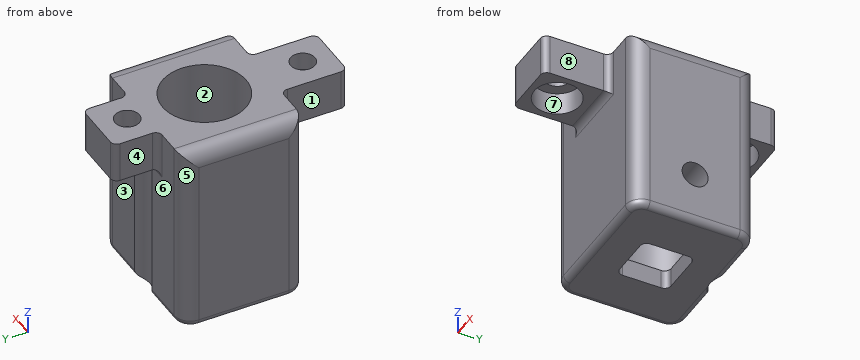
```python
from build123d import *

# Parameters (mm, degrees)
SKETCH1_W                                      = 23
SKETCH1_H                                      = 19
SKETCH1_W_2                                    = 8
SKETCH1_H_2                                    = 8
TOP_DEPTH                                      = 3
SKETCH1_4_W                                    = 23
SKETCH1_4_H                                    = 19
SKETCH1_4_R                                    = 6.5
BODY_DEPTH                                     = 29.83
TABS_START                                     = 23.48
SKETCH1_6_W                                    = 9
SKETCH1_6_H                                    = 7
SKETCH1_6_H_2                                  = 10.3075
TABS_DEPTH                                     = 6.35
F_36_0_1065_DIA_SET_SCREW_D                    = 4.0386
F_36_0_1065_DIA_SET_SCREW_DEPTH                = 4.826
F_36_0_1065_DIA_SET_SCREW_TIP                  = 1.213317848
CBORE_FOR_6_SOCKET_HEAD_CAP_SCREW1_D           = 3.7973
CBORE_FOR_6_SOCKET_HEAD_CAP_SCREW1_CBORE_D     = 7.14502
CBORE_FOR_6_SOCKET_HEAD_CAP_SCREW1_CBORE_DEPTH = 26.9851886
FILLET4_R                                      = 2.5
FILLET5_R                                      = 1


with BuildPart() as part:
    # Sketch1 → Top (new body)
    with BuildSketch(Plane.XY):
        Rectangle(SKETCH1_W, SKETCH1_H)
        Rectangle(SKETCH1_W_2, SKETCH1_H_2, mode=Mode.SUBTRACT)
    extrude(amount=TOP_DEPTH)

    # Sketch1<4> → Body (add)
    with BuildSketch(Plane.XY):
        Rectangle(SKETCH1_4_W, SKETCH1_4_H)
        Circle(SKETCH1_4_R, mode=Mode.SUBTRACT)
    extrude(amount=BODY_DEPTH)

    # Sketch1<6> → Tabs (add)
    with BuildSketch(Plane.XY.offset(TABS_START)):
        with Locations((0, 13)):
            Rectangle(SKETCH1_6_W, SKETCH1_6_H)
        with Locations((0, -14.65375)):
            Rectangle(SKETCH1_6_W, SKETCH1_6_H_2)
    extrude(amount=TABS_DEPTH)

    # #36 (0.1065) Dia. Set Screw
    with Locations(Plane(origin=(11.5, 0, 0), x_dir=(0, 0, -1), z_dir=(1, 0, 0))):
        with Locations((-8, 0)):
            Hole(F_36_0_1065_DIA_SET_SCREW_D / 2, depth=F_36_0_1065_DIA_SET_SCREW_DEPTH)
            with Locations((0, 0, -(F_36_0_1065_DIA_SET_SCREW_DEPTH + F_36_0_1065_DIA_SET_SCREW_TIP / 2))):  # 118° drill point
                Cone(0, F_36_0_1065_DIA_SET_SCREW_D / 2, F_36_0_1065_DIA_SET_SCREW_TIP, mode=Mode.SUBTRACT)

    # CBORE for #6 Socket Head Cap Screw1 (through all)
    with Locations(Plane(origin=(0, 12, 0), x_dir=(-1, 0, 0), z_dir=(0, 0, -1))):
        with Locations((0, 0), (0, -27.3035)):
            CounterBoreHole(CBORE_FOR_6_SOCKET_HEAD_CAP_SCREW1_D / 2, CBORE_FOR_6_SOCKET_HEAD_CAP_SCREW1_CBORE_D / 2, CBORE_FOR_6_SOCKET_HEAD_CAP_SCREW1_CBORE_DEPTH)

    # Fillet4
    fillet4_edges = [part.edges().sort_by_distance(p)[0] for p in [
        (-11.5, 9.5, 14.915),
        (-11.5, -9.5, 14.915),
        (11.5, -9.5, 14.915),
        (11.5, 9.5, 14.915),
        (-11.5, 0, 29.83),
        (11.5, 0, 29.83),
    ]]
    fillet(fillet4_edges, radius=FILLET4_R)

    # Fillet5
    fillet5_edges = [part.edges().sort_by_distance(p)[0] for p in [
        (-11.5, 0, 0),
        (11.5, 0, 0),
        (0, -9.5, 0),
        (-5.776012118, 9.5, 0),
        (10.767766953, 8.767766953, 0),
        (10.767766953, -8.767766953, 0),
        (-10.767766953, -8.767766953, 0),
        (-10.767766953, 8.767766953, 0),
        (-4, 4, 1.5),
        (-4, -4, 1.5),
        (4, -4, 1.5),
        (4, 4, 1.5),
        (-4.5, 16.5, 26.655),
        (-3.526012118, 9.5, 23.48),
        (-4.5, 9.5, 26.655),
        (4.5, 9.5, 26.655),
        (4.5, 16.5, 26.655),
        (4.5, -9.5, 26.655),
        (-4.5, -9.5, 26.655),
        (-4.5, -19.8075, 26.655),
        (4.5, -19.8075, 26.655),
        (0, -9.5, 23.48),
        (5.776012118, 9.5, 0),
    ]]
    fillet(fillet5_edges, radius=FILLET5_R)


solid = part.part
```
Could you check a few things on this model? Use its own coordinates, in mm. Face numbers are marked on the shaded views. A direction names the side the tool comes from. Give positions to 0.01 mm unless a question says otherwise; leave off trailing zeros. Order: outer loops, then holes, each group sorted by start corner. A loop starts at its lowest first (then second) coordinate and runs counter-clockwise, first axis right, second up.
Q1. I'm going to push flat-ended pins straight in: P1, Ø10, axis at x = -0.5, y = -15, coming from the -Z side; P2, Ø2, axis at x = 2, z = 10.5, coming from the +Y side; P3, Ø0.9, axis at x = -1, z = 1, coming from the +Y side (3 decimals); P4, Ø12, axis at y = -16, z = 16, coming from the +X side. Where does each tip first touch, or does it pass through?
Q2. Suppose I cut it at D-D, the plane x = -7.5. Write out the boundary of the cut face in (y, z).
Q3. We'd pull the mould along X, two halves only. Please class the marked faces 5, 6, 7 and 8: +X half, -X half, draft (parallel to the pull), parting line (faces both ways), or undercut.
Q4. Suppose I cut it at C-C, the plane y = 0. Write out the boundary of the cut face in (x, z), and give its area (3 significant figures).
Q5. Suppose I cut it at B-B, the plane z = 14. Write out the boundary of the cut face in (x, y).
Q6. For the marked faces 1, 2, 3 and 4, which set-ups out of +Z, -Z, +X, -X, +Y, -Y let a thin tool reach every point of the face, with its end or its side?
Q7. Suppose I cut it at A-A, the plane x = 0. Count the separate pieces of the cut face and the enclosed holes in it, and give its area (3 significant figures).
Q8. If I drill on line 1 along Y through (x, z) = (0, 28.9); line 2 along Y through (x, z) = (0, 24.6); line 3 along Y through (x, z) = (0, 12), over which ranges is the centre line in solid material (lowest first)?
Solution:
1. P1: stops at z = 23.35
1. P2: stops at y = 9.5
1. P3: stops at y = 8.735
1. P4: passes through
2. outline: (-9.5, 1) arc R1 ccw to (-8.5, 0) - (8.5, 0) arc R1 ccw to (9.5, 1) - (9.5, 29.83) - (-9.5, 29.83) - close
3. face 5: -X half
3. face 6: draft
3. face 7: undercut
3. face 8: +X half
4. outline: (-11.5, 1) arc R1 ccw to (-10.5, 0) - (-4, 0) - (-4, 3) - (-6.5, 3) - (-6.5, 29.83) - (-9, 29.83) arc R2.5 ccw to (-11.5, 27.33) - close; (4, 0) - (10.5, 0) arc R1 ccw to (11.5, 1) - (11.5, 5.98) - (6.67, 5.98) - (6.5, 6.27) - (6.5, 3) - (4, 3) - close; (6.5, 9.73) - (6.67, 10.02) - (11.5, 10.02) - (11.5, 27.33) arc R2.5 ccw to (9, 29.83) - (6.5, 29.83) - close
4. area: 290 mm2
5. outline: (-11.5, -7) arc R2.5 ccw to (-9, -9.5) - (9, -9.5) arc R2.5 ccw to (11.5, -7) - (11.5, 7) arc R2.5 ccw to (9, 9.5) - (2.55, 9.5) arc R3.57 cw to (-2.55, 9.5) - (-9, 9.5) arc R2.5 ccw to (-11.5, 7) - close; hole circle Ø13 at (0, 0)
6. face 1: +Z, -Z, -X, -Y
6. face 2: +Z
6. face 3: -Z, +X, +Y
6. face 4: +Z, -Z, -X, +Y
7. separate pieces: 4
7. enclosed holes: 0
7. area: 207 mm2
8. line 1: y = -19.81 to -17.2, -13.4 to -6.5, 6.5 to 10.1, 13.9 to 16.5
8. line 2: y = -19.81 to -18.88, -11.73 to -6.5, 6.5 to 8.43, 15.57 to 16.5
8. line 3: y = -9.5 to -6.5, 6.5 to 8.43
